CAD build for the part. Positions are in the model's coordinates, mm. A direction names the side the tool comes from. Round coordinates to 2 decimals unless told otherwise and drop trailing zeros. Write each loop counter-clockwise with the first axis right and the second up, starting at its lowest first coordinate (ties: lowest second). Pieces come first, ordered by that corner, then holes. Notation, with made-up numbers: (39, 82) - (89, 82) arc R31 cw to (89, 117) - close; hole circle Ø7 at (-36, -21). An arc over 180 degrees is marked (long way). Put each result on its own line as item: value. Start each with the question number.
Item 1: Drill centre lines: line 1 (X direction, y = -56.5, z = 2.5) (3 decimals); line 2 (Y direction, x = 10.5, z = 18.5); line 3 (Z direction, x = -5, y = -38.5) (3 decimals). Where is each one in solid material? Low to high. Write a range as from..to.
Item 2: Pin check, flat tips, straight feed: pin 1 Ø15 at (x, y) = (77, -10.5) entering from -Z; pin 2 Ø4 at (y, z) = (-28, 45.5) entering from +X; pin 3 Ø8.5 at (y, z) = (13.5, 14.5) entering from -X (3 decimals); pin 4 Ø3 at (x, z) = (82.5, 48.5) entering from +Y. Stop position of each tip, or through.
Item 3: Cut at B-B (x = 93). Give the cut face in (y, z) (3 decimals).
Item 4: 3-axis set-ups, long thin cutter, end or side, ignore diameter. For faces 4 (the flat face through (46, -25.4, 42)), 5 (the flat face through (22.225, 17, 18)), 6 (the cylindrical face through (31.94, -16.79, 51.17)), 7 (the flat face through (41.275, -1, 4)): which of +Z, -Z, +X, -X, +Y, -Y reach the whole face in a straight line?
Item 5: Cut at A-A (x = 65). Give the cut face in (y, z) (1 decimal), and give its area (3 significant figures).
Item 6: Mould opens along X. For faces 1 (the flat face through (-41.275, -1, 0)), 2 (the flat face through (60, -2, 61.925)), 3 (the flat face through (60, 2, 42.875)) say: released by +X, released by -X, zero draft, split by the parting line, or undercut.
```python
from build123d import *

# Parameters (mm, degrees)
F1_DEPTH = 63.5
F0_W     = 25.4
F0_H     = 19.05
F2_DEPTH = 25.4
F3_DEPTH = 7.9375


with BuildPart() as f1:
    # F0 (on Front) → F1 (new body, symmetric)
    with BuildSketch(Plane.XZ):
        Polygon((-41.275, -9.525), (41.275, -9.525), (41.275, 9.525), (22.225, 9.525), (-41.275, 9.525), align=None)
    extrude(amount=F1_DEPTH, both=True)

    # F0 (on Front) → F2 (join, symmetric)
    with BuildSketch(Plane.XZ):
        with Locations((73.025, 52.4002)):
            Rectangle(F0_W, F0_H)
        with BuildLine():
            Line((22.225, 9.525), (41.275, 9.525))
            Line((41.275, 9.525), (41.275, 27.0002))
            ThreePointArc((41.275, 27.0002), (45.9246798487, 38.2255201513), (57.15, 42.8752))
            Line((57.15, 42.8752), (60.325, 42.8752))
            Line((60.325, 42.8752), (60.325, 61.9252))
            Line((60.325, 61.9252), (57.15, 61.9252))
            add(Edge.make_bspline(
                [(54.9392255171, 61.8551580574), (55.7011340945, 61.8864647718), (56.4386307378, 61.9096636569), (57.15, 61.9252)],
                knots=[108.4110637299, 108.4110637299, 108.4110637299, 108.4110637299, 111.5045361635, 111.5045361635, 111.5045361635, 111.5045361635], degree=3))
            ThreePointArc((54.9392255171, 61.8551580574), (31.6846615591, 50.9015004477), (22.225, 27.0002))
            Line((22.225, 27.0002), (22.225, 9.525))
        make_face()
    extrude(amount=F2_DEPTH, both=True)

    # F0 (on Front) → F3 (join, symmetric)
    with BuildSketch(Plane.XZ):
        with BuildLine():
            add(Edge.make_bspline(
                [(-41.275, 9.525), (-28.4448499709, 49.7031577837), (28.2380600433, 60.7580109912), (54.9392255171, 61.8551580574)],
                knots=[0, 0, 0, 0, 108.4110637299, 108.4110637299, 108.4110637299, 108.4110637299], degree=3))
            Line((-41.275, 9.525), (22.225, 9.525))
            Line((22.225, 9.525), (22.225, 27.0002))
            ThreePointArc((22.225, 27.0002), (31.6846615591, 50.9015004477), (54.9392255171, 61.8551580574))
        make_face()
    extrude(amount=F3_DEPTH, both=True)

    # F0 (on Front) → F4 (revolve)
    with BuildSketch(Plane.XZ):
        Polygon((85.725, 61.9252), (85.725, 42.8752), (85.725, 38.1), (111.125, 38.1), (111.125, 66.675), (85.725, 66.675), align=None)
    revolve(axis=Axis((85.725, 0, 52.3875), (0, 0, 1)))


solid = f1.part
```
Output values:
1. line 1: -41.275..41.275
1. line 2: -7.94..7.94
1. line 3: -9.525..9.525
2. pin 1: z = 38.1
2. pin 2: through
2. pin 3: x = 22.225
2. pin 4: y = 25.4
3. outline: (-24.336, 38.1) - (24.336, 38.1) - (24.336, 66.675) - (-24.336, 66.675) - close
4. face 4: +Z, +X, -X, -Y
4. face 5: +Z, -X, +Y
4. face 6: +Z, -X, -Y
4. face 7: -Z, +X, +Y, -Y
5. outline: (-25.4, 42.9) - (-14.7, 42.9) - (-14.7, 38.1) - (14.7, 38.1) - (14.7, 42.9) - (25.4, 42.9) - (25.4, 61.9) - (14.7, 61.9) - (14.7, 66.7) - (-14.7, 66.7) - (-14.7, 61.9) - (-25.4, 61.9) - close
5. area: 1,250 mm2
6. face 1: released by -X
6. face 2: zero draft
6. face 3: undercut
